Drawing for the job (mm, zero at the part's lowest x, y, z). A direction names the side the tool comes from. Coordinates: 2 decimals unless noted, no trailing zeros. Loops run counter-clockwise (first coordinate to the right, second up) from the corner with the lowest first, then second, coordinate; pieces in that order, holes last.
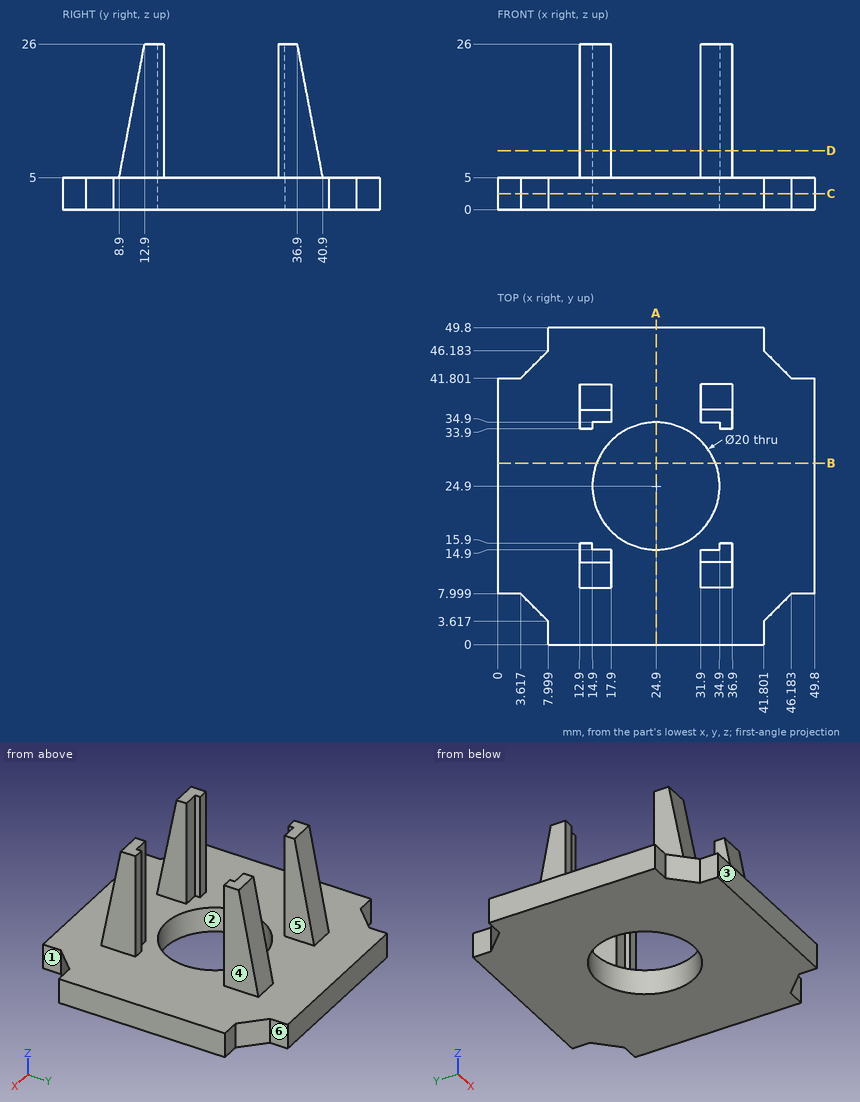
Q1. Saw through at A-A (x = 24.9). List the corners of the cut face in (y, z), plus the area to 3 significant figures.
Q2. Saw through at B-B (y = 28.5). List the corners of the cut face in (x, z).
Q3. Saw through at C-C (z = 2.5). List the corners of the cut face in (x, y), plus the area to 3 significant figures.
Q4. Drop flat-ended pins along their axis: P1, Ø8, axis at x = 20.5, y = 33.5, coming from the -Z side; P2, Ø1.5, axis at x = 34, z = 6.5, coming from the -Y side; P3, Ø1.8, axis at x = 2.5, z = 1.5, coming from the -Y side; P4, Ø1.1, axis at x = 47.5, z = 2.5, coming from the +Y side. Give the stop position or say it passes through.
Q5. Probe line 1 (X direction, y = 11, z = 11); line 2 (Y direction, x = 24.9, z = 2.55); line 3 (Z direction, x = 17, y = 3.5). List the from-to ranges inside material, lowest first.
Q6. Tool access for the marked faces 4, 5 and 6: list every direction of +Z, -Z, +X, -X, +Y, -Y with a clear straight run to the whole face (end or side of a thin tool).
Q7. Mould opens along X. For the marked faces 1, 2 and 3 say: released by +X, released by -X, zero draft, split by the parting line, or undercut.
Q8. Saw through at D-D (z = 9.25). List the corners of the cut face in (x, y), plus the area to 3 significant figures.
Checked values:
1. outline: (0, 0) - (14.9, 0) - (14.9, 5) - (0, 5) - close; (34.9, 0) - (49.8, 0) - (49.8, 5) - (34.9, 5) - close
1. area: 149 mm2
2. outline: (0, 0) - (15.57, 0) - (15.57, 5) - (0, 5) - close; (34.23, 0) - (49.8, 0) - (49.8, 5) - (34.23, 5) - close
3. outline: (0, 8) - (3.62, 8) - (8, 3.62) - (8, 0) - (41.8, 0) - (41.8, 3.62) - (46.18, 8) - (49.8, 8) - (49.8, 41.8) - (46.18, 41.8) - (41.8, 46.18) - (41.8, 49.8) - (8, 49.8) - (8, 46.18) - (3.62, 41.8) - (0, 41.8) - close; hole circle Ø20 at (24.9, 24.9)
3. area: 1,950 mm2
4. P1: stops at z = 0
4. P2: stops at y = 9.04
4. P3: stops at y = 8
4. P4: stops at y = 41.8
5. line 1: x = 12.9 to 17.9, 31.9 to 36.9
5. line 2: y = 0 to 14.9, 34.9 to 49.8
5. line 3: z = 0 to 5
6. face 4: +Z, +X, +Y, -Y
6. face 5: +Z, +Y, -Y
6. face 6: +Z, -Z, +X, +Y
7. face 1: released by +X
7. face 2: undercut
7. face 3: zero draft
8. outline: (12.9, 9.71) - (17.9, 9.71) - (17.9, 14.9) - (14.9, 14.9) - (14.9, 15.9) - (12.9, 15.9) - close; (12.9, 33.9) - (14.9, 33.9) - (14.9, 34.9) - (17.9, 34.9) - (17.9, 40.09) - (12.9, 40.09) - close; (31.9, 9.71) - (36.9, 9.71) - (36.9, 15.9) - (34.9, 15.9) - (34.9, 14.9) - (31.9, 14.9) - close; (31.9, 34.9) - (34.9, 34.9) - (34.9, 33.9) - (36.9, 33.9) - (36.9, 40.09) - (31.9, 40.09) - close
8. area: 112 mm2
